Part print with two shaded views. Sizes in mm from the minimum x, y, z corner. Give positions to 0.01 mm unless a question says otherwise; leave off trailing zeros. Order: outer loops, then holes, each group sorted by start corner. A loop starts at its lowest first (then second) coordinate and runs counter-clockwise, first axis right, second up.
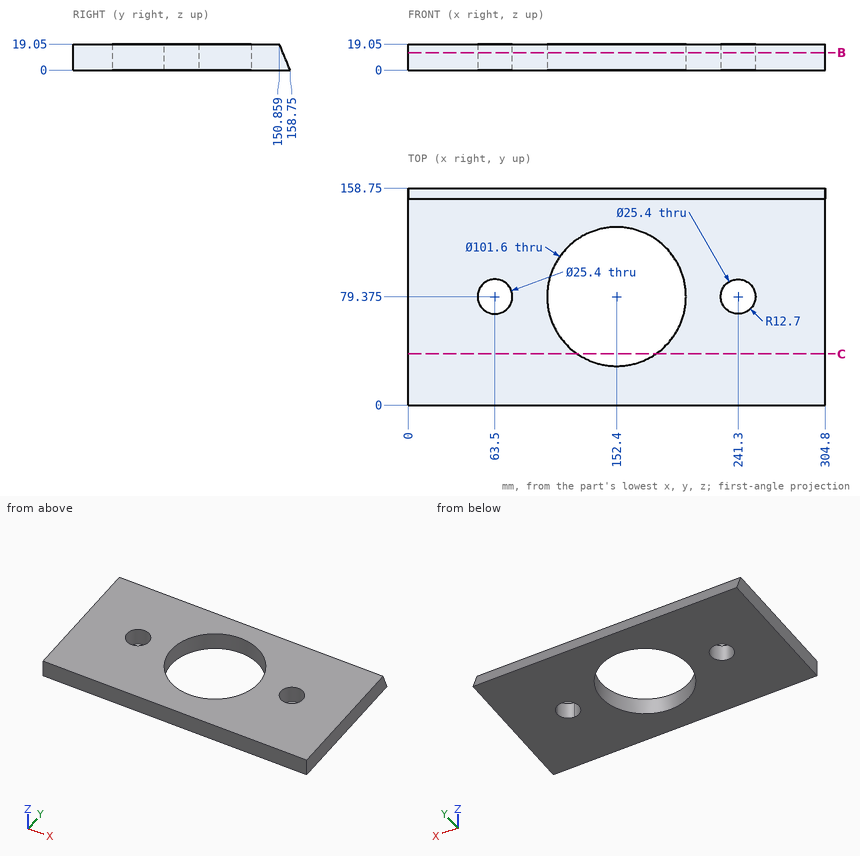
Item 1: Drop flat-ended pins along their axis: pin 1 Ø1.5 at (x, y) = (262.5, 37.5) entering from -Z; pin 2 Ø20.5 at (x, y) = (241.3, 79.375) entering from -Z; pin 3 Ø6 at (x, z) = (265.5, 14.5) entering from +Y. Give the stop position or say it passes through.
Item 2: Wall check: L1, parallel to X at y = 70, z = 17; L2, parallel to X at y = 61.5, z = 6.5; L3, parallel to Y at x = 159.5, z = 17. Give the ranges that are in metal, low to high.
Item 3: Slice it at B-B (z = 12.75). Give the cut face in (x, y) (1 decimal), and give its area (3 significant figures).
Item 4: Slice it at C-C (y = 37.5). Give the cut face in (x, z).
A:
1. pin 1: stops at z = 0
1. pin 2: passes through
1. pin 3: stops at y = 153.99
2. L1: x = 0 to 54.93, 72.07 to 102.47, 202.33 to 232.73, 249.87 to 304.8
2. L2: x = 0 to 104.85, 199.95 to 304.8
2. L3: y = 0 to 29.07, 129.68 to 151.71
3. outline: (0, 0) - (304.8, 0) - (304.8, 153.5) - (0, 153.5) - close; hole circle Ø25.4 at (63.5, 79.4); hole circle Ø101.6 at (152.4, 79.4); hole circle Ø25.4 at (241.3, 79.4)
3. area: 37,700 mm2
4. outline: (0, 0) - (123.64, 0) - (123.64, 19.05) - (0, 19.05) - close; (181.16, 0) - (304.8, 0) - (304.8, 19.05) - (181.16, 19.05) - close
